```python
from build123d import *

# Parameters (mm, degrees)
BOSS_EXTRUDE1_DEPTH = 30
SKETCH2_R           = 7.5
CUT_EXTRUDE1_DEPTH  = 30
SKETCH5_R           = 1.5
CUT_EXTRUDE2_DEPTH  = 30


with BuildPart() as part:
    # Sketch1 → Boss-Extrude1 (new body)
    with BuildSketch(Plane(origin=(0, 0, 0), x_dir=(0, 0, -1), z_dir=(1, 0, 0))):
        Polygon((0, 0), (18, 0), (18, 33), (21, 33), (21, -2), (0, -2), align=None)
    extrude(amount=BOSS_EXTRUDE1_DEPTH)

    # Sketch2 → Cut-Extrude1 (cut)
    with BuildSketch(Plane.XY.offset(-18)):
        with Locations((15, 22)):
            Circle(SKETCH2_R)
    extrude(amount=-CUT_EXTRUDE1_DEPTH, mode=Mode.SUBTRACT)

    # Sketch5 → Cut-Extrude2 (cut)
    with BuildSketch(Plane(origin=(0, 0, 0), x_dir=(1, 0, 0), z_dir=(0, 1, 0))):
        with Locations((5, 3)):
            Circle(SKETCH5_R)
        with Locations((17, 3)):
            Circle(SKETCH5_R)
        with Locations((29, 3)):
            Circle(SKETCH5_R)
        with Locations((17, 15)):
            Circle(SKETCH5_R)
        with Locations((29, 15)):
            Circle(SKETCH5_R)
        with Locations((5, 15)):
            Circle(SKETCH5_R)
    extrude(amount=-CUT_EXTRUDE2_DEPTH, mode=Mode.SUBTRACT)


solid = part.part
```
CAD build for the part. Positions are in the model's coordinates, mm. A direction names the side the tool comes from. Round coordinates to 2 decimals unless told otherwise and drop trailing zeros. Order: outer loops, then holes, each group sorted by start corner. A loop starts at its lowest first (then second) coordinate and runs counter-clockwise, first axis right, second up. Notation, with made-up numbers: (6, 18) - (43, 18) arc R17 cw to (43, 45) - close; hole circle Ø6 at (46, -19.75). An arc over 180 degrees is marked (long way). Answer in a Markdown table with one row per item. Add a question column.
(1) Mould opens along X. For faces 1 (the face through (27.5, -1, -15)), 2 (the face through (30, 16, -19)), 3 (the face through (15, 12, -21)) say: +X half, -X half, draft (parallel to the pull), parting line (faces both ways), or undercut.
(2) Band-saw the part on C-C on x = 15. List the corners of the cut face in (y, z), and give its area (3 significant figures).
(3) Band-saw the part on D-D on y = 21. List the corners of the cut face in (x, z).
(4) Band-saw the part on B-B on z = -3. List the corners of the cut face in (x, y).
(5) Drop flat-ended pins along their axis: pin 1 Ø6 at (x, z) = (25, -7) entering from +Y; pin 2 Ø8 at (x, y) = (21, 15) entering from +Z. Give the stop position or say it passes through.
(6) Band-saw the part on A-A on x = 6. List the corners of the cut face in (y, z).
(7) 3-axis set-ups, long thin cutter, end or side, ignore diameter. For faces 4 (the face through (15, 13, -18)), 5 (the face through (30, -1, -9)): which of +Z, -Z, +X, -X, +Y, -Y reach the whole face in a straight line?
(8) Probe L1, parallel to Z at x = 29, y = -0.6; L2, parallel to X at y = -1.6, z = -3; L3, parallel to Y at x = 2.5, z = -16.75. List the from-to ranges inside material, lowest first. Write a range as [from, to].
Data:
| question | item | result |
|---|---|---|
| 1 | face 1 | undercut |
| 1 | face 2 | +X half |
| 1 | face 3 | draft |
| 2 | outline | (-2, -21) - (14.5, -21) - (14.5, -18) - (0, -18) - (0, 0) - (-2, 0) - close; (29.5, -21) - (33, -21) - (33, -18) - (29.5, -18) - close |
| 2 | area | 96.0 mm^2 |
| 3 | outline | (0, -21) - (7.57, -21) - (7.57, -18) - (0, -18) - close; (22.43, -21) - (30, -21) - (30, -18) - (22.43, -18) - close |
| 4 | outline | (0, -2) - (3.5, -2) - (3.5, 0) - (0, 0) - close; (6.5, -2) - (15.5, -2) - (15.5, 0) - (6.5, 0) - close; (18.5, -2) - (27.5, -2) - (27.5, 0) - (18.5, 0) - close |
| 5 | pin 1 | stops at y = 0 |
| 5 | pin 2 | stops at z = -18 |
| 6 | outline | (-2, -21) - (33, -21) - (33, -18) - (0, -18) - (0, -16.12) - (-2, -16.12) - close; (-2, -13.88) - (0, -13.88) - (0, -4.12) - (-2, -4.12) - close; (-2, -1.88) - (0, -1.88) - (0, 0) - (-2, 0) - close |
| 7 | face 4 | +Z, +X, -X, +Y |
| 7 | face 5 | +Z, -Z, +X, +Y, -Y |
| 8 | L1 | z = [-21, -16.5], [-13.5, -4.5], [-1.5, 0] |
| 8 | L2 | x = [0, 3.5], [6.5, 15.5], [18.5, 27.5] |
| 8 | L3 | y = [-2, 0] |
